Verification items for the finished model (mm, model axes). A direction names the side the tool comes from. Give positions to 0.01 mm unless a question says otherwise; leave off trailing zeros. Order: outer loops, then holes, each group sorted by start corner. A loop starts at its lowest first (then second) coordinate and runs counter-clockwise, first axis right, second up. Notation, with made-up numbers: (55.25, 41.5) - (75.25, 41.5) arc R24 ccw to (75.25, 57.5) - close; hole circle Ø11 at (37, 71.25). An arc over 180 degrees is marked (long way). Answer as a JSON object with one key per item and string values. Group by question number.
(1) Section check B-B (z = -18). Record the boundary of the cut face in (x, y) (1 decimal), then the cut area to 3 significant figures.
(2) Section check D-D (x = -7.5). Record the boundary of the cut face in (y, z) (1 decimal).
(3) Section check C-C (y = -54). Record the boundary of the cut face in (x, z).
(4) Thickness scan on line 1 (X direction, y = -66, z = -18); line 2 (X direction, y = -32, z = 39); line 3 (Z direction, x = 36, y = -61.5). Record the ranges inside material, lowest first.
(5) Depth check by flat-ended pin: pin 1 Ø8 at (x, z) = (-56.5, 16.5) entering from +Y (3 decimals); pin 2 Ø6 at (x, z) = (32.5, -13.5) entering from -Y; pin 3 Ø3.5 at (x, y) = (-28.5, -64) entering from +Z. Enter the tip coordinate at first touch or a pass-through.
(6) Access from +Z, -Z, +X, -X, +Y, -Y to the whole of each face (thin tool, end or side, straight path). Record for faces 4 (the face through (-3, -36, -28.311)), 5 (the face through (35, -1.225, -8)), 6 (the face through (69.674, -16.192, 37.139)), 7 (the face through (69, -67, -3.102)), 8 (the face through (-0.848, -67, 15)).
(7) Mould release check, pull along X, two halves, no side actions. Record for faces 1 (the face through (67.282, -67, -15)), 2 (the face through (-73, -67, -3.102)), 3 (the face through (70.457, -37, 5)): +X half, -X half, draft (parallel to the pull), parting line (faces both ways), or undercut.
(8) Section check A-A (x = 59). Record the boundary of the cut face in (y, z) (1 decimal), then the cut area to 3 significant figures.
Solid Edge part; units mm, degrees
sketch "Sketch1" plane through (33.0178, -67.9125, -28.311) normal (0, 0, -1) x (1, 0, 0)
  line L0 (-107.3551, -66.6879) -> (-107.3551, 4.73)
  line L1 (-107.3551, 4.73) -> (37.4389, 4.73)
  line L2 (37.4389, 4.73) -> (37.4389, -66.6879)
  line L3 (37.4389, -66.6879) -> (-107.3551, -66.6879)
extrude "bottom" add sketch "Sketch1" against normal blind 1.5875
sketch "Sketch2" plane through (-4.9364, -1.2246, -1.8296) normal (0, 1, 0) x (-1, 0, 0)
  line L0 (-75.3931, 19.2386) -> (-75.3931, 0.7937)
  line L1 (-75.3931, 0.7937) -> (-75.3931, -26.4814)
  line L2 (-75.3931, -26.4814) -> (69.4009, -26.4814)
  line L3 (69.4009, 0.7937) -> (69.4009, -26.4814)
  line L4 (69.4009, 19.2386) -> (69.4009, 0.7937)
  line L5 (-75.3931, 19.2386) -> (69.4009, 19.2386)
extrude "back" add sketch "Sketch2" along normal blind 1.5875
sketch "Sketch3" plane through (33.0178, -60.6425, 33.925) normal (0, 1, 0) x (-1, 0, 0)
  line L0 (35.5, 24.664) -> (107.2281, 24.664)
  line L1 (107.2281, -30.75) -> (107.2281, 24.664)
  line L2 (107.2281, -30.75) -> (107.2281, -62.236)
  line L3 (107.2281, -62.236) -> (-37.3119, -62.236)
  line L4 (-37.3119, -62.236) -> (-37.3119, -30.75)
  line L5 (-37.3119, 24.664) -> (-37.3119, -30.75)
  line L6 (35.5, 24.664) -> (-37.3119, 24.664)
extrude "front_sub_panel" add sketch "Sketch3" along normal blind 1.5875
extrude "front_panel" [suppressed]
sketch "Sketch4" plane through (-3.0325, -72.0075, 33.8361) normal (1, 0, 0) x (0, 0, -1)
  line L0 (-24.7529, -0.635) -> (36.7471, -0.635)
  line L1 (36.7471, -0.635) -> (36.7471, 1.143)
  line L2 (36.7471, 1.143) -> (62.1471, 1.143)
  line L3 (62.1471, 12.9525) -> (62.1471, 1.143)
  line L4 (-24.7529, 12.9525) -> (62.1471, 12.9525)
  line L5 (-24.7529, 12.9525) -> (-24.7529, -0.635)
extrude "Protrusion1" add sketch "Sketch4" along normal up to vertex (2.1844 mm away)
sketch "Sketch5" plane through (-1.9403, -36.9336, -26.7235) normal (0, 0, 1) x (1, 0, 0)
  line L0 (-69.222, -35.7089) -> (-69.222, -22.1214)
  line L1 (-69.222, -22.1214) -> (-72.397, -22.1214)
  line L2 (-72.397, -22.1214) -> (-72.397, -35.7089)
  line L3 (-72.397, -35.7089) -> (-69.222, -35.7089)
  line L4 (69.222, -22.1214) -> (72.397, -22.1214)
  line L5 (72.397, -22.1214) -> (72.397, -35.7089)
  line L6 (72.397, -35.7089) -> (69.222, -35.7089)
  line L7 (69.222, -35.7089) -> (69.222, -22.1214)
extrude "sub_panel_sides" add sketch "Sketch5" along normal blind 23.622
sketch "Sketch6" plane through (70.4567, -36.1398, -5.451) normal (1, 0, 0) x (0, 1, 0)
  line L0 (3.8491, 61.7751) -> (36.5027, 22.86)
  line L1 (36.5027, 22.86) -> (36.5027, -22.86)
  line L2 (36.5027, -22.86) -> (-24.5027, -22.86)
  line L3 (-24.5027, 8.626) -> (-24.5027, -22.86)
  line L4 (-24.5027, 64.04) -> (-24.5027, 8.626)
  line L5 (-22.9152, 64.04) -> (-24.5027, 64.04)
  line L6 (3.8491, 61.7751) -> (-22.9152, 64.04)
extrude "ExtrudedProtrusion_7" add sketch "Sketch6" against normal blind 1.5875
sketch "Sketch7" plane through (-74.3373, -36.1398, -5.451) normal (-1, 0, 0) x (0, -1, 0)
  line L0 (22.9152, 64.04) -> (24.5027, 64.04)
  line L1 (-3.8491, 61.7751) -> (22.9152, 64.04)
  line L2 (-3.8491, 61.7751) -> (-36.5027, 22.86)
  line L3 (-36.5027, 22.86) -> (-36.5027, -22.86)
  line L4 (-36.5027, -22.86) -> (24.5027, -22.86)
  line L5 (24.5027, 8.626) -> (24.5027, -22.86)
  line L6 (24.5027, 64.04) -> (24.5027, 8.626)
extrude "ExtrudedProtrusion_8" add sketch "Sketch7" against normal blind 1.5875
sketch "Sketch8" plane through (-1.9403, -59.055, 15.9327) normal (0, 1, 0) x (-1, 0, 0)
  line L0 (-32.9495, -39.7988) -> (-32.9495, 1.4762)
  line L1 (-32.9495, 1.4762) -> (70.8095, 1.4762)
  line L2 (70.8095, 1.4762) -> (70.8095, -39.7988)
  line L3 (70.8095, -39.7988) -> (-32.9495, -39.7988)
extrude "Cutout1" cut sketch "Sketch8" along normal up to next
Solutions:
{
 "1": {"outline": "(-74.3, -72.6) - (-71.2, -72.6) - (-71.2, -60.6) - (-3, -60.6) - (-3, -70.9) - (-0.8, -70.9) - (-0.8, -60.6) - (67.3, -60.6) - (67.3, -72.6) - (70.5, -72.6) - (70.5, 0.4) - (31, 0.4) - (31, -1.2) - (68.9, -1.2) - (68.9, -59.1) - (-72.7, -59.1) - (-72.7, 0.4) - (-74.3, 0.4) - close", "area": "577 mm2"},
 "2": {"outline": "(-72.6, -28.3) - (0.4, -28.3) - (0.4, -23.9) - (-1.2, -23.9) - (-1.2, -26.7) - (-59.1, -26.7) - (-59.1, 58.6) - (-60.6, 58.6) - (-60.6, -26.7) - (-72.6, -26.7) - close"},
 "3": {"outline": "(-74.34, -28.31) - (70.46, -28.31) - (70.46, 58.16) - (68.87, 58.16) - (68.87, -26.72) - (-72.75, -26.72) - (-72.75, 58.16) - (-74.34, 58.16) - close"},
 "4": {"line 1": "x = -74.34 to -71.16, -3.03 to -0.85, 67.28 to 70.46", "line 2": "x = -74.34 to -72.75, 68.87 to 70.46", "line 3": "z = -28.31 to -26.72"},
 "5": {"pin 1": "stops at y = -59.055", "pin 2": "stops at y = -60.64", "pin 3": "stops at z = -26.72"},
 "6": {"face 4": "-Z, +X, -X, +Y, -Y", "face 5": "+Z", "face 6": "+Z, +X, -X, +Y", "face 7": "+Z, +X, -Y", "face 8": "+Z, -Y"},
 "7": {"face 1": "undercut", "face 2": "draft", "face 3": "+X half"},
 "8": {"outline": "(-72.6, -28.3) - (0.4, -28.3) - (0.4, 17.4) - (-1.2, 17.4) - (-1.2, -26.7) - (-59.1, -26.7) - (-59.1, 58.6) - (-60.6, 58.6) - (-60.6, -26.7) - (-72.6, -26.7) - close", "area": "321 mm2"}
}
